Part model, mm, in its own coordinate system. Face numbers are marked on the shaded views. A direction names the side the tool comes from. Coordinates: 2 decimals unless noted, no trailing zeros. Order: outer loops, then holes, each group sorted by start corner. A loop starts at its lowest first (then second) coordinate and runs counter-clockwise, first axis right, second up.
from build123d import *

# Parameters (mm, degrees)
SKETCH1_W           = 25.5
SKETCH1_H           = 24
BOSS_EXTRUDE1_DEPTH = 1.3
SKETCH2_W           = 25.5
SKETCH2_H           = 5.4
BOSS_EXTRUDE2_DEPTH = 4
SKETCH3_R           = 2
CUT_EXTRUDE1_DEPTH  = 4
SKETCH4_R           = 2
CUT_EXTRUDE2_DEPTH  = 4


with BuildPart() as part:
    # Sketch1 → Boss-Extrude1 (new body)
    with BuildSketch(Plane.XY):
        with Locations((14.577148508, 8.992218626)):
            Rectangle(SKETCH1_W, SKETCH1_H)
    extrude(amount=BOSS_EXTRUDE1_DEPTH)

    # Sketch2 → Boss-Extrude2 (add)
    with BuildSketch(Plane.XY.offset(1.3)):
        with Locations((14.577148508, 8.992218626)):
            Rectangle(SKETCH2_W, SKETCH2_H)
    extrude(amount=BOSS_EXTRUDE2_DEPTH)

    # Sketch3 → Cut-Extrude1 (cut)
    with BuildSketch(Plane.XY.offset(1.3)):
        with Locations((22.327148508, 16.492218626)):
            Circle(SKETCH3_R)
        with Locations((6.827148508, 16.492218626)):
            Circle(SKETCH3_R)
    extrude(amount=-CUT_EXTRUDE1_DEPTH, mode=Mode.SUBTRACT)

    # Sketch4 → Cut-Extrude2 (cut)
    with BuildSketch(Plane.XY.offset(1.3)):
        with Locations((6.827148508, 1.492218626)):
            Circle(SKETCH4_R)
        with Locations((22.327148508, 1.492218626)):
            Circle(SKETCH4_R)
    extrude(amount=-CUT_EXTRUDE2_DEPTH, mode=Mode.SUBTRACT)


solid = part.part
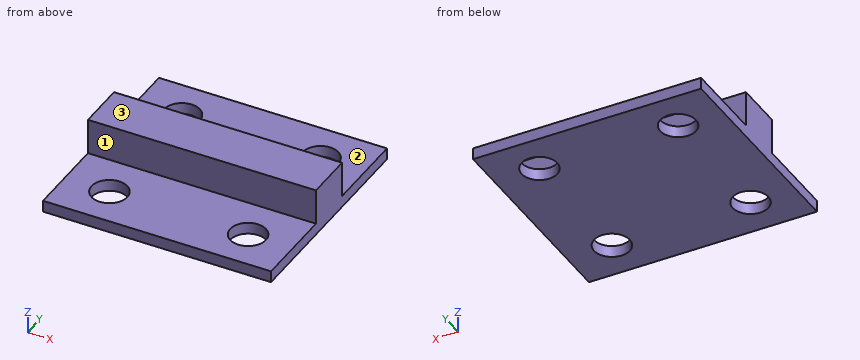
Q1. Cut at B-B on y = 2.5. Write the cut outline in (x, z).
Results list:
outline: (1.83, 0) - (5.1, 0) - (5.1, 1.3) - (1.83, 1.3) - close; (8.55, 0) - (20.6, 0) - (20.6, 1.3) - (8.55, 1.3) - close; (24.05, 0) - (27.33, 0) - (27.33, 1.3) - (24.05, 1.3) - close
Q2. Cut at D-D on z = 3. Write the cut outline in (x, y), and give its area (3 significant figures).
Results list:
outline: (1.83, 6.29) - (27.33, 6.29) - (27.33, 11.69) - (1.83, 11.69) - close
area: 138 mm2
Q3. Which spindle directions (+Z, -Z, +X, -X, +Y, -Y) get a long thin tool onto all of the face, cutting with end or side? Do the marked faces 1, 2 and 3. Say none if no direction does.
Results list:
face 1: +Z, +X, -X, -Y
face 2: +Z, +X, -X, +Y
face 3: +Z, +X, -X, +Y, -Y
Q4. Wall check: line 1 along Y through (x, z) = (9.5, 1.8); line 2 along Y through (x, z) = (21.5, 0.3); line 3 along Z through (x, y) = (24.5, 14.5). Give the ranges that are in metal, low to high.
Results list:
line 1: y = 6.29 to 11.69
line 2: y = -3.01 to -0.33, 3.31 to 14.67, 18.31 to 20.99
line 3: z = 0 to 1.3
Q5. Cut at A-A on x = 23.5. Write the cut outline in (y, z), and give its area (3 significant figures).
Results list:
outline: (-3.01, 0) - (-0.13, 0) - (-0.13, 1.3) - (-3.01, 1.3) - close; (3.11, 0) - (14.87, 0) - (14.87, 1.3) - (11.69, 1.3) - (11.69, 5.3) - (6.29, 5.3) - (6.29, 1.3) - (3.11, 1.3) - close; (18.11, 0) - (20.99, 0) - (20.99, 1.3) - (18.11, 1.3) - close
area: 44.4 mm2
Q6. Pin check, flat tips, straight feed: pin 1 Ø6.5 at (x, y) = (22.33, 16.49) entering from +Z; pin 2 Ø10 at (x, y) = (12.5, 3) entering from +Z; pin 3 Ø1.2 at (x, z) = (16, 2.5) entering from -Y. Stop position of each tip, or through.
Results list:
pin 1: stops at z = 1.3
pin 2: stops at z = 5.3
pin 3: stops at y = 6.29
Q7. Cut at C-C on x = 14. Write the cut outline in (y, z), and give its area (3 significant figures).
Results list:
outline: (-3.01, 0) - (20.99, 0) - (20.99, 1.3) - (11.69, 1.3) - (11.69, 5.3) - (6.29, 5.3) - (6.29, 1.3) - (-3.01, 1.3) - close
area: 52.8 mm2
